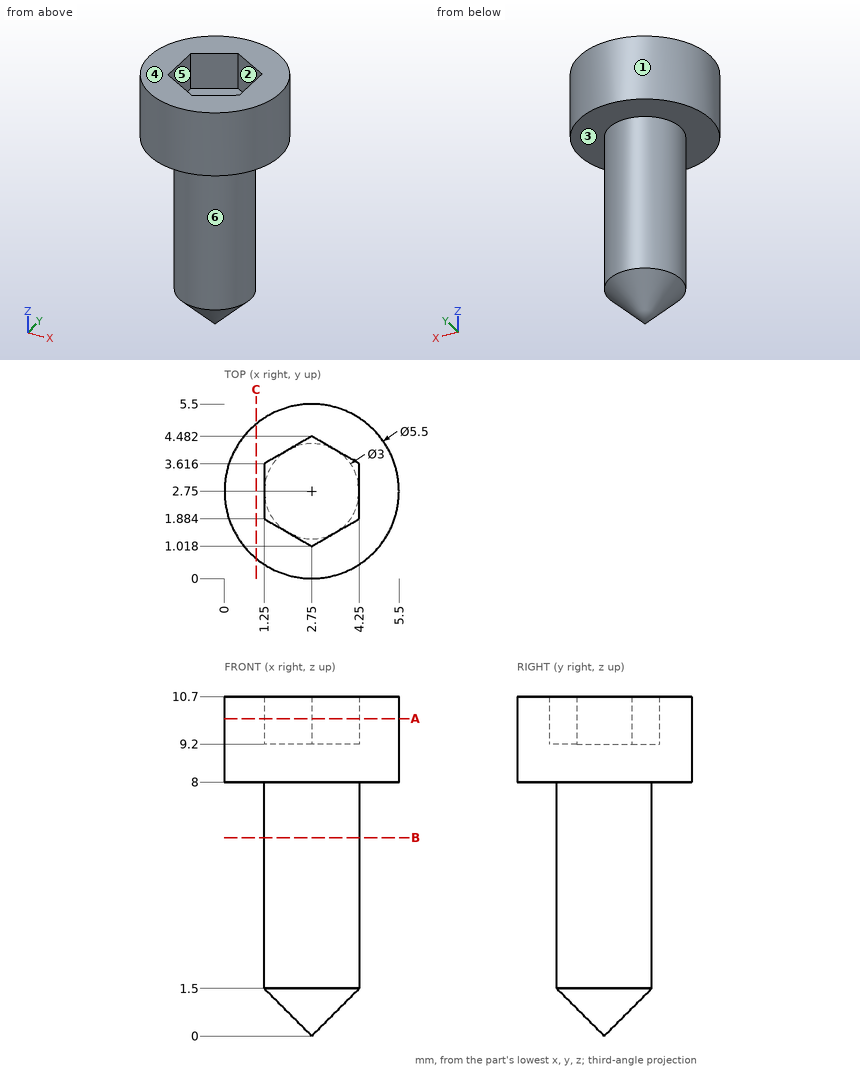
Verification items for this drawing (mm, ordinates from the low corner). A direction names the side the tool comes from. Coordinates: 2 decimals unless noted, no trailing zeros. Write each loop counter-clockwise with the first axis right and the second up, starting at its lowest first coordinate (ties: lowest second). Pieces come first, ordered by that corner, then holes. Notation, with made-up numbers: M -22,63.25 L 24,63.25 A25 ccw 24,101.25 Z; hole C 44,78 d6. An arc over 180 degrees is marked long. Answer as a JSON object with one key per item and string values. Group by question number.
(1) Material ranges on line 1 (Z direction, x = 3.9, y = 1.1); line 2 (X direction, y = 3.4, z = 10.25); line 3 (X direction, y = 2.7, z = 3), recorded low to high.
(2) Release check for a two-part mould opening along X. For the marked faces 1, 2 and 3 record: +X half, -X half, draft (parallel to the pull), parting line (faces both ways), or undercut.
(3) Tool access check on the marked faces 4, 5 and 6. Record the directions out of +Z, -Z, +X, -X, +Y, -Y that give a thin tool (end or side, any length) a straight path to the whole face; none if there is none.
(4) Cross-section at B-B, the plane z = 6.25. Record the cut outline in (x, y), and give its area (3 significant figures).
(5) Gauge pin test, flat end, axial feed: pin 1 (2 mm diameter, centred on x = 1.5, z = 1.5, fed in from -Y). Record the tip position at first contact, or that the pin passes through.
(6) Cross-section at C-C, the plane x = 1. Record the cut outline in (y, z), and give its area (3 significant figures).
(7) Cross-section at A-A, the plane z = 10. Record the cut outline in (x, y), and give its area (3 significant figures).
Reply:
{
 "1": {"line 1": "8 to 10.7", "line 2": "0.08 to 1.25, 4.25 to 5.42", "line 3": "1.25 to 4.25"},
 "2": {"face 1": "parting line", "face 2": "undercut", "face 3": "draft"},
 "3": {"face 4": "+Z, +X, -X, +Y, -Y", "face 5": "+Z", "face 6": "-Z"},
 "4": {"outline": "C 2.75,2.75 d3", "area": "7.07 mm²"},
 "5": {"pin 1": "y = 1.27"},
 "6": {"outline": "M 0.63,8 L 4.87,8 L 4.87,10.7 L 0.63,10.7 Z", "area": "11.5 mm²"},
 "7": {"outline": "C 2.75,2.75 d5.5; hole M 1.25,1.88 L 2.75,1.02 L 4.25,1.88 L 4.25,3.62 L 2.75,4.48 L 1.25,3.62 Z", "area": "16.0 mm²"}
}
